Read the model definition and answer for the solid it produces. Units are mm, in the model's axes. Face numbers are marked on the shaded views. A direction names the side the tool comes from. Coordinates: 2 decimals unless noted, no trailing zeros. Loops run counter-clockwise (first coordinate to the right, second up) from the corner with the lowest first, then second, coordinate; pieces in that order, holes last. Notation, with made-up numbers: (13, 78.5) - (47, 78.5) arc R24 cw to (47, 95.5) - close; hole circle Ø8 at (82.25, 16). An arc over 180 degrees is marked (long way). Use one line per item in the form item = value. Start each with the question number.
1) A cutting plane is placed at A-A (z = 31.75). Give the vertices of the cut face in (x, y) (3 decimals).
2) A cutting plane is placed at D-D (y = 32). Give the vertices of the cut face in (x, z), and give its area (3 significant figures).
3) A cutting plane is placed at C-C (y = 12). Give the vertices of the cut face in (x, z) (3 decimals).
4) Each of these flat-tipped pins is pushed along its axis until it touches: P1, Ø6, axis at y = 42.5, z = 42, coming from the +X side; P2, Ø6, axis at x = 8, y = 48, coming from the -Z side; P3, Ø13.5, axis at x = -13, y = 21, coming from the +Z side; P4, Ø22, axis at x = 36, z = 20.5, coming from the +Y side. Where does it stop, or does it pass through?
5) Which of the six approach directions +Z, -Z, +X, -X, +Y, -Y give full straight-line access (tool end or side, diameter ignored) to the marked faces 1, 2 and 3?
6) A cutting plane is placed at B-B (x = 44.45). Give the vertices of the cut face in (y, z) (3 decimals), and give its area (3 significant figures).
7) Consider line 1 (X direction, y = 14.5, z = 31.75) (3 decimals); line 2 (X direction, y = 8, z = 31); line 3 (X direction, y = 14, z = 50.5). Determine where each line is inside the solid, lowest interval first.
8) The mould has two halves that part along X. Classify the marked faces 4, 5, 6 and 7: released by +X, released by -X, zero draft, split by the parting line, or undercut.
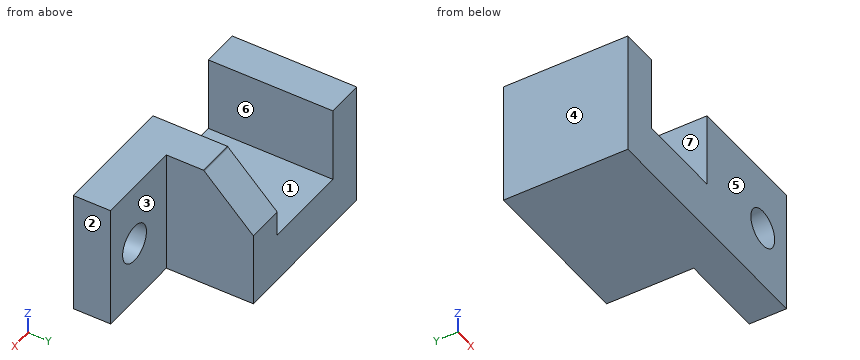
Autodesk Inventor part; units mm, degrees
ref_plane "YZ Plane" through (0, 0, 0) normal (1, 0, 0) x (0, 1, 0)
ref_plane "XZ Plane" through (0, 0, 0) normal (0, 1, 0) x (-1, 0, 0)
ref_plane "XY Plane" through (0, 0, 0) normal (0, 0, 1) x (1, 0, 0)
sketch "Sketch1" plane through (0, 0, 0) normal (0, 0, 1) x (1, 0, 0)
  line L0 (0, 0) -> (0, 63.5)
  line L1 (0, 63.5) -> (19.05, 63.5)
  line L2 (0, 0) -> (63.5, 0)
  line L3 (63.5, 0) -> (63.5, 19.05)
  line L4 (63.5, 19.05) -> (19.05, 19.05)
  line L5 (19.05, 19.05) -> (19.05, 63.5)
  dimension "d3" = 63.5
  dimension "d6" = 19.05
  dimension "d7" = 63.5
  dimension "d8" = 19.05
  dimension "d9" = 44.45
  dimension "d10" = 44.45
extrude "Extrusion1" add sketch "Sketch1" along normal blind 63.5
sketch "Sketch2" plane through (0, 63.5, 0) normal (0, 1, 0) x (1, 0, 0)
  line L0 (0, 0) -> (-63.5, 0)
  line L1 (-63.5, 0) -> (-63.5, -63.5)
  line L2 (-63.5, -63.5) -> (-44.45, -63.5)
  line L3 (0, 0) -> (0, -63.5)
  line L4 (0, -6.0479) -> (0, -25.0979)
  line L5 (0, -25.0979) -> (-44.45, -25.0979)
  line L6 (-44.45, -25.0979) -> (-44.45, -63.5)
  dimension "d19" = 63.5
  dimension "d20" = 63.5
  dimension "d21" = 19.05
  dimension "d22" = 19.05
  dimension "d23" = 38.4021
  dimension "d24" = 44.45
extrude "Extrusion2" add sketch "Sketch2" against normal blind 63.5
sketch "Sketch3" plane through (19.05, 19.05, 0) normal (0, 1, 0) x (1, 0, 0)
  line L0 (44.45, 0) -> (44.45, -63.5)
  line L1 (-82.55, 0) -> (44.45, 0)
  circle A0 centre (25.4, -31.75) radius 9.525
  point P0 (-19.05, 0)
  dimension "d29" = 19.05
extrude "Extrusion3" cut sketch "Sketch3" along normal blind 63.5 and the other way blind 31.75
sketch "Sketch4" plane through (19.05, 19.05, 0) normal (1, 0, 0) x (0, 0, -1)
  line L0 (-63.5, 44.45) -> (-25.0979, 44.45)
  line L1 (-63.5, 44.45) -> (-38.1, 44.45)
  line L2 (-38.1, 44.45) -> (-63.1713, 19.3817)
  line L3 (-63.1713, 19.3817) -> (-63.5, 19.0531)
  line L4 (-63.5, 44.45) -> (-63.5, -19.05)
  point P0 (0, -19.05)
  dimension "d34" = 25.4
extrude "Extrusion4" cut sketch "Sketch4" against normal blind 50.8
properties part number "INVENTOR_TUT" material "Polypropylene"
Found:
q1.outline = (-63.5, 0) - (-44.45, 0) - (-44.45, 63.5) - (-63.5, 63.5) - close; (0, 0) - (34.925, 0) - (34.925, 19.05) - (19.05, 19.05) - (19.05, 63.5) - (0, 63.5) - close; (53.975, 0) - (63.5, 0) - (63.5, 19.05) - (53.975, 19.05) - close
q2.outline = (-63.5, 0) - (19.05, 0) - (19.05, 63.5) - (0, 63.5) - (0, 25.1) - (-44.45, 25.1) - (-44.45, 63.5) - (-63.5, 63.5) - close
q2.area = 3,530 mm^2
q3.outline = (-63.5, 0) - (63.5, 0) - (63.5, 63.5) - (0, 63.5) - (0, 25.098) - (-44.45, 25.098) - (-44.45, 63.5) - (-63.5, 63.5) - close; hole circle Ø19.05 at (44.45, 31.75)
q4.P1 = 19.05
q4.P2 = 0
q4.P3 = 25.1
q4.P4 = 19.05
q5.face_1 = +Z, +Y, -Y
q5.face_2 = +Z, -Z, +X, +Y, -Y
q5.face_3 = +Z, -Z, +X, +Y
q6.outline = (0, 0) - (19.05, 0) - (19.05, 22.225) - (0, 22.225) - close; (0, 41.275) - (19.05, 41.275) - (19.05, 63.5) - (0, 63.5) - close
q6.area = 847 mm^2
q7.line_1 = -63.5 to -44.45, 0 to 34.925, 53.975 to 63.5
q7.line_2 = -63.5 to -44.45, 0 to 34.95, 53.95 to 63.5
q7.line_3 = -63.5 to -44.45, 0 to 63.5
q8.face_4 = released by -X
q8.face_5 = zero draft
q8.face_6 = undercut
q8.face_7 = undercut
